The listing builds one solid part. Answer for the finished solid, in the listing's coordinates (mm). A direction names the side the tool comes from. Coordinates: 2 decimals unless noted, no trailing zeros. Order: outer loops, then holes, each group sorted by start corner. A loop starts at its lowest first (then second) coordinate and runs counter-clockwise, first axis right, second up.
from build123d import *

# Parameters (mm, degrees)
SKETCH_1_R          = 1.25
SKETCH_1_R_2        = 1
EXTRUDE_1_DEPTH     = 2
SKETCH_4_W          = 15.5
SKETCH_4_H          = 22
CUT_EXTRUDE_1_DEPTH = 2
FILLET_2_R          = 2.5
FILLET_3_R          = 5
SKETCH_6_W          = 16
SKETCH_6_H          = 32
CUT_EXTRUDE_3_DEPTH = 10


with BuildPart() as part:
    # 草圖1 → 填料-伸長1 (new body)
    with BuildSketch(Plane.XY):
        with BuildLine():
            Line((-17.216213198, 10.1625), (13.283786802, 10.1625))
            Line((13.283786802, 10.1625), (13.283786802, -21.8375))
            Line((13.283786802, -21.8375), (-17.216213198, -21.8375))
            Line((-17.216213198, -21.8375), (-19.716213198, -21.8375))
            Line((-19.716213198, -21.8375), (-25.716213198, -21.8375))
            Line((-25.716213198, -21.8375), (-25.716213198, -15.8375))
            ThreePointArc((-25.716213198, -15.8375), (-24.716213198, -14.8375), (-25.716213198, -13.8375))
            Line((-25.716213198, -13.8375), (-27.716213198, -13.8375))
            Line((-27.716213198, -13.8375), (-27.716213198, -9.8375))
            Line((-27.716213198, -9.8375), (-25.716213198, -9.8375))
            ThreePointArc((-25.716213198, -9.8375), (-24.716213198, -8.8375), (-25.716213198, -7.8375))
            Line((-25.716213198, -7.8375), (-25.716213198, -3.8375))
            ThreePointArc((-25.716213198, -3.8375), (-24.716213198, -2.8375), (-25.716213198, -1.8375))
            Line((-25.716213198, -1.8375), (-27.716213198, -1.8375))
            Line((-27.716213198, -1.8375), (-27.716213198, 2.1625))
            Line((-27.716213198, 2.1625), (-25.716213198, 2.1625))
            ThreePointArc((-25.716213198, 2.1625), (-24.716213198, 3.1625), (-25.716213198, 4.1625))
            Line((-25.716213198, 4.1625), (-25.716213198, 10.1625))
            Line((-25.716213198, 10.1625), (-21.716213198, 10.1625))
            Line((-21.716213198, 10.1625), (-17.216213198, 10.1625))
        make_face()
        with Locations((-19.216213198, 7.6625)):
            Circle(SKETCH_1_R, mode=Mode.SUBTRACT)
        with Locations((-19.216213198, -19.3375)):
            Circle(SKETCH_1_R, mode=Mode.SUBTRACT)
        with Locations((10.783786802, -19.3375)):
            Circle(SKETCH_1_R, mode=Mode.SUBTRACT)
        with Locations((10.783786802, 7.6625)):
            Circle(SKETCH_1_R, mode=Mode.SUBTRACT)
        with Locations((-23.716213198, -11.8375)):
            Circle(SKETCH_1_R_2, mode=Mode.SUBTRACT)
        with Locations((-23.716213198, 0.1625)):
            Circle(SKETCH_1_R_2, mode=Mode.SUBTRACT)
    extrude(amount=EXTRUDE_1_DEPTH)

    # 草圖4 → 除料-伸長1 (cut)
    with BuildSketch(Plane(origin=(0, 0, 0), x_dir=(-1, 0, 0), z_dir=(0, 0, -1))):
        with Locations((-5.533786802, -5.8375)):
            Rectangle(SKETCH_4_W, SKETCH_4_H)
    extrude(amount=-CUT_EXTRUDE_1_DEPTH, mode=Mode.SUBTRACT)

    # 圓角2
    fillet_2_edges = [part.edges().sort_by_distance(p)[0] for p in [
        (13.283786802, -16.8375, 1),
        (13.283786802, 5.1625, 1),
    ]]
    fillet(fillet_2_edges, radius=FILLET_2_R)

    # 圓角3
    fillet_3_edges = [part.edges().sort_by_distance(p)[0] for p in [
        (-2.216213198, 5.1625, 1),
        (-2.216213198, -16.8375, 1),
    ]]
    fillet(fillet_3_edges, radius=FILLET_3_R)

    # 草圖6 → 除料-伸長3 (cut)
    with BuildSketch(Plane(origin=(0, 0, 0), x_dir=(-1, 0, 0), z_dir=(0, 0, -1))):
        with Locations((-5.283786802, -5.8375)):
            Rectangle(SKETCH_6_W, SKETCH_6_H)
    extrude(amount=-CUT_EXTRUDE_3_DEPTH, mode=Mode.SUBTRACT)


solid = part.part
(1) Find section C-C on z = 1.65. Determine the outline of the cut face in (x, y).
(2) Find section B-B on y = 8. Determine the outline of the cut face in (x, z), then the cut area to 3 significant figures.
(3) Given pin 1 Ø1 at (y, z) = (6.5, 1) entering from -X; pin 2 Ø1.2 at (x, y) = (-23.72, 0.16) entering from +Z; pin 3 Ø0.6 at (x, z) = (-27, 1.5) entering from +Y; pin 4 Ø1 at (x, z) = (-27, 1) entering from -Y, each flat-ended and moving along its own axis, determine where each tip first touches the part or whether it passes through.
(4) Find section D-D on x = -19.75. Determine the outline of the cut face in (y, z).
(5) Find the intervals of material crossed by probe 1 along Y at (x, z) = (-24, 0.45); probe 2 along Y at (x, z) = (-20, 0.5); probe 3 along X at (y, z) = (7, 1.3), in increasing order.
(6) The mould has two halves that part along X. Classify faces 4 (the flat face through (-27, -1.838, 1)), 5 (the cylindrical face through (-24.716, -8.859, 0.986)), 6 (the cylindrical face through (-20.208, 6.902, 0.986)): pulls with the +X half, pulls with the -X half, needs draft (parallel to the pull), parting line crosses it, or undercut.
(7) A tool of negligible diameter and unlimited length cuts with its end or side. For faces 1 (the flat face through (-27, -9.838, 1)), 2 (the flat face through (-27, 2.162, 1)), 3 (the flat face through (-27, -13.838, 1)), from which of +Z, -Z, +X, -X, +Y, -Y can it reach the whole face along a straight path? Write none if from no direction.
(8) Find section A-A on x = -25.25. Determine the outline of the cut face in (y, z).
Resolved:
1. outline: (-27.72, -13.84) - (-25.72, -13.84) arc R1 cw to (-25.72, -15.84) - (-25.72, -21.84) - (-2.72, -21.84) - (-2.72, 10.16) - (-25.72, 10.16) - (-25.72, 4.16) arc R1 cw to (-25.72, 2.16) - (-27.72, 2.16) - (-27.72, -1.84) - (-25.72, -1.84) arc R1 cw to (-25.72, -3.84) - (-25.72, -7.84) arc R1 cw to (-25.72, -9.84) - (-27.72, -9.84) - close; hole circle Ø2 at (-23.72, -11.84); hole circle Ø2 at (-23.72, 0.16); hole circle Ø2.5 at (-19.22, -19.34); hole circle Ø2.5 at (-19.22, 7.66)
2. outline: (-25.72, 0) - (-20.42, 0) - (-20.42, 2) - (-25.72, 2) - close; (-18.01, 0) - (-2.72, 0) - (-2.72, 2) - (-18.01, 2) - close
2. area: 41.2 mm2
3. pin 1: stops at x = -25.72
3. pin 2: passes through
3. pin 3: stops at y = 2.16
3. pin 4: stops at y = -13.84
4. outline: (-21.84, 0) - (-20.47, 0) - (-20.47, 2) - (-21.84, 2) - close; (-18.21, 0) - (6.53, 0) - (6.53, 2) - (-18.21, 2) - close; (8.79, 0) - (10.16, 0) - (10.16, 2) - (8.79, 2) - close
5. probe 1: y = -21.84 to -12.8, -10.88 to -0.8, 1.12 to 10.16
5. probe 2: y = -21.84 to -20.31, -18.36 to 6.69, 8.64 to 10.16
5. probe 3: x = -25.72 to -20.28, -18.16 to -2.72
6. face 4: needs draft
6. face 5: pulls with the -X half
6. face 6: undercut
7. face 1: +Z, -Z, -X
7. face 2: +Z, -Z, -X, +Y
7. face 3: +Z, -Z, -X, -Y
8. outline: (-21.84, 0) - (-15.72, 0) - (-15.72, 2) - (-21.84, 2) - close; (-13.95, 0) - (-9.72, 0) - (-9.72, 2) - (-13.95, 2) - close; (-7.95, 0) - (-3.72, 0) - (-3.72, 2) - (-7.95, 2) - close; (-1.95, 0) - (2.28, 0) - (2.28, 2) - (-1.95, 2) - close; (4.05, 0) - (10.16, 0) - (10.16, 2) - (4.05, 2) - close
